Read the model definition and answer for the solid it produces. Units are mm, in the model's axes. A direction names the side the tool comes from. Give positions to 0.01 mm unless a question says otherwise; leave off trailing zeros. Order: outer loops, then holes, each group sorted by start corner. A loop starts at its lowest first (then second) coordinate and runs counter-clockwise, first axis right, second up. Notation, with made-up numbers: (52.5, 55) - (107.5, 55) arc R25 cw to (107.5, 80) - close; hole circle Ø9 at (61, 47). An arc over 180 degrees is marked (long way). Return JSON: item names as keys, results as strings.
```python
from build123d import *

# Parameters (mm, degrees)
BOSS_EXTRUDE2_DEPTH    = 6
FILLET1_R              = 1
LPATTERN1_COUNT        = 3
LPATTERN1_PITCH        = 37.5
FILLET1_OF_LPATTERN1_R = 1
SKETCH3_W              = 6
SKETCH3_H              = 12
BOSS_EXTRUDE3_DEPTH    = 6
SKETCH4_W              = 8
SKETCH4_H              = 6
CUT_EXTRUDE2_DEPTH     = 7
LPATTERN2_COUNT        = 2
LPATTERN2_PITCH        = 37.5
BOSS_EXTRUDE4_START    = -112.5
SKETCH3_2_W            = 6
SKETCH3_2_H            = 12
BOSS_EXTRUDE4_DEPTH    = 6
SKETCH5_W              = 6
SKETCH5_H              = 22.5
BOSS_EXTRUDE5_DEPTH    = 6


with BuildPart() as part:
    # Sketch2 → Boss-Extrude2 (new body)
    with BuildSketch(Plane(origin=(0, 0, 0), x_dir=(0, 0, -1), z_dir=(1, 0, 0))):
        Polygon((-18.75, 123.5), (-18.75, 107.5), (-18.75, -107.5), (18.75, -107.5), (18.75, 107.5), (18.75, 123.5), (12, 123.5), (11, 113.5), (4, 113.5), (4, 107.5), (-4, 107.5), (-4, 113.5), (-11, 113.5), (-12, 123.5), align=None)
    boss_extrude2 = extrude(amount=BOSS_EXTRUDE2_DEPTH)

    # Fillet1
    fillet1_edges = [part.edges().sort_by_distance(p)[0] for p in [
        (3, 113.5, -4),
        (3, 123.5, -12),
        (3, 123.5, 12),
        (3, 113.5, 4),
        (3, 107.5, 4),
        (3, 107.5, -4),
    ]]
    fillet(fillet1_edges, radius=FILLET1_R)

    # LPattern1: Boss-Extrude2 ×3
    with Locations(*[(0, 0, i * LPATTERN1_PITCH) for i in range(1, LPATTERN1_COUNT)]):
        add(boss_extrude2)

    # Fillet1 of LPattern1
    fillet1_of_lpattern1_edges = [part.edges().sort_by_distance(p)[0] for p in [
        (3, 113.5, 33.5),
        (3, 123.5, 25.5),
        (3, 123.5, 49.5),
        (3, 113.5, 41.5),
        (3, 107.5, 41.5),
        (3, 107.5, 33.5),
        (3, 113.5, 71),
        (3, 123.5, 63),
        (3, 123.5, 87),
        (3, 113.5, 79),
        (3, 107.5, 79),
        (3, 107.5, 71),
    ]]
    fillet(fillet1_of_lpattern1_edges, radius=FILLET1_OF_LPATTERN1_R)

    # Sketch3 → Boss-Extrude3 (add)
    with BuildSketch(Plane(origin=(0, 0, -18.75), x_dir=(-1, 0, 0), z_dir=(0, 0, -1))):
        with Locations((-3, 97.5)):
            Rectangle(SKETCH3_W, SKETCH3_H)
        with Locations((-3, -81.5)):
            Rectangle(SKETCH3_W, SKETCH3_H)
        with Locations((-3, 8)):
            Rectangle(SKETCH3_W, SKETCH3_H)
    extrude(amount=BOSS_EXTRUDE3_DEPTH)

    # Sketch4 → Cut-Extrude2 (cut, through all)
    with BuildSketch(Plane(origin=(0, 0, 0), x_dir=(0, 0, -1), z_dir=(1, 0, 0))):
        with Locations((-18.75, 104.5)):
            Rectangle(SKETCH4_W, SKETCH4_H)
    cut_extrude2 = extrude(amount=CUT_EXTRUDE2_DEPTH, mode=Mode.SUBTRACT)

    # LPattern2: Cut-Extrude2 ×2
    with Locations(*[(0, 0, i * LPATTERN2_PITCH) for i in range(1, LPATTERN2_COUNT)]):
        add(cut_extrude2, mode=Mode.SUBTRACT)

    # Sketch3_2 → Boss-Extrude4 (add)
    with BuildSketch(Plane(origin=(0, 0, -18.75), x_dir=(-1, 0, 0), z_dir=(0, 0, -1)).offset(BOSS_EXTRUDE4_START)):
        with Locations((-3, 97.5)):
            Rectangle(SKETCH3_2_W, SKETCH3_2_H)
        with Locations((-3, -81.5)):
            Rectangle(SKETCH3_2_W, SKETCH3_2_H)
        with Locations((-3, 8)):
            Rectangle(SKETCH3_2_W, SKETCH3_2_H)
    extrude(amount=-BOSS_EXTRUDE4_DEPTH)

    # Sketch5 → Boss-Extrude5 (add)
    with BuildSketch(Plane.XZ.offset(107.5)):
        with Locations((3, 15)):
            Rectangle(SKETCH5_W, SKETCH5_H)
        with Locations((3, 60)):
            Rectangle(SKETCH5_W, SKETCH5_H)
    extrude(amount=BOSS_EXTRUDE5_DEPTH)


solid = part.part
```
Q1. Given pin 1 (1 mm diameter, centred on x = 2.5, y = 41, fed in from +Z); pin 2 (1.8 mm diameter, centred on x = 2.5, y = 113.5, fed in from -Z); pin 3 (3 mm diameter, centred on x = 2.5, z = 34.5, fed in from -Y), each flat-ended and moving along its own axis, determine where each tip first touches the part or whether it passes through.
Values:
{"pin 1": "stops at z = 93.75", "pin 2": "stops at z = -18.75", "pin 3": "stops at y = -107.5"}
Q2. Determine the mould class of faces 5 (the flat face through (3, -97, 93.75)), 6 (the flat face through (3, 53, 93.75)), 7 (the flat face through (2.96, 118.11, 63.54)) for opening direction Y: released by +Y, released by -Y, zero draft, split by the parting line, or undercut.
Values:
{"face 5": "zero draft", "face 6": "undercut", "face 7": "released by +Y"}
Q3. A cutting plane is placed at D-D (z = -16). Write down the section's boundary in (x, y), and give its area (3 significant figures).
Values:
{"outline": "(0, -107.5) - (6, -107.5) - (6, 123.5) - (0, 123.5) - close", "area": "1,390 mm²"}
Q4. A cutting plane is placed at B-B (x = 3.65). Give the number of separate pieces and of enclosed holes in the cut face, and give its area (3 significant figures).
Values:
{"separate pieces": "1", "enclosed holes": "2", "area": "25,800 mm²"}
Q5. A cutting plane is placed at C-C (y = -39). Write down the section's boundary in (x, z).
Values:
{"outline": "(0, -18.75) - (6, -18.75) - (6, 93.75) - (0, 93.75) - close"}
Q6. Consider L1, parallel to Y at x = 4.6, z = 75.5; L2, parallel to Y at x = 1.6, z = 65; L3, parallel to Z at x = 1.35, y = -12.5. Determine where each line is inside the solid, lowest interval first.
Values:
{"L1": "y = -107.5 to 107.5", "L2": "y = -113.5 to 113.5", "L3": "z = -18.75 to 93.75"}
Q7. A cutting plane is placed at A-A (z = 55). Write down the section's boundary in (x, y).
Values:
{"outline": "(0, -113.5) - (6, -113.5) - (6, 101.5) - (0, 101.5) - close; (0, 107.5) - (6, 107.5) - (6, 123.5) - (0, 123.5) - close"}
Q8. For faces 1 (the flat face through (3, -75.5, -22)), 2 (the flat face through (3, 107.5, 75)), 3 (the flat face through (3, 104, 60.25)), 4 (the flat face through (3, 91.5, 97)), determine the directions among +Z, -Z, +X, -X, +Y, -Y from which every point of the face is accessible in a straight line to the end or side of a thin tool.
Values:
{"face 1": "-Z, +X, -X", "face 2": "+X, -X, +Y", "face 3": "+X, -X", "face 4": "+Z, +X, -X"}
